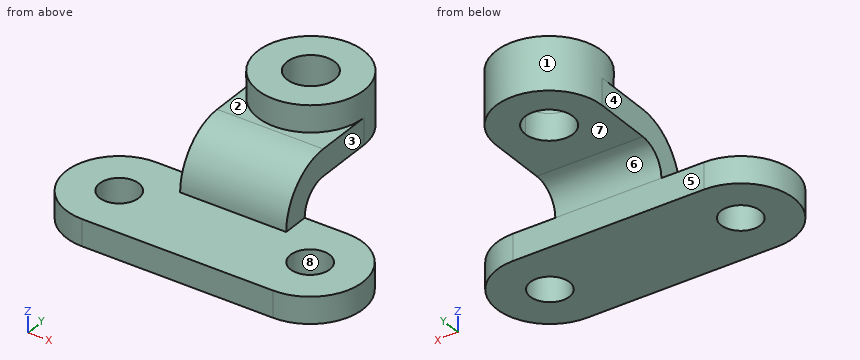
```python
from build123d import *
from build123d.topology import SkipClean

# Parameters (mm, degrees)
SKETCH1_R           = 18.5
BOSS_EXTRUDE1_DEPTH = 25
BOSS_EXTRUDE2_START = 100
SKETCH1_3_R         = 50
SKETCH1_3_R_2       = 22.5
BOSS_EXTRUDE2_DEPTH = 50
BOSS_EXTRUDE3_DEPTH = 50
CUT_EXTRUDE1_DEPTH  = 241.052077683


with BuildPart() as part:
    # Sketch1 → Boss-Extrude1 (new body)
    with BuildSketch(Plane.XY):
        with BuildLine():
            Line((-90, -50), (90, -50))
            ThreePointArc((90, -50), (140, 0), (90, 50))
            Line((90, 50), (-90, 50))
            ThreePointArc((-90, 50), (-140, 0), (-90, -50))
        make_face()
        with Locations((-90, 0)):
            Circle(SKETCH1_R, mode=Mode.SUBTRACT)
        with Locations((90, 0)):
            Circle(SKETCH1_R, mode=Mode.SUBTRACT)
    extrude(amount=BOSS_EXTRUDE1_DEPTH)



with BuildPart() as body_2:
    # Sketch1<3> → Boss-Extrude2 (new body)
    with BuildSketch(Plane.XY.offset(BOSS_EXTRUDE2_START)):
        with Locations((0, 130)):
            Circle(SKETCH1_3_R)
        with Locations((0, 130)):
            Circle(SKETCH1_3_R_2, mode=Mode.SUBTRACT)
    extrude(amount=-BOSS_EXTRUDE2_DEPTH)


with BuildPart() as part_1:
    add(part.part)

    add(body_2.part)  # Boss-Extrude3 merges body 2
    # Sketch2 → Boss-Extrude3 (add, symmetric)
    with BuildSketch(Plane(origin=(0, 0, 0), x_dir=(0, 0, -1), z_dir=(1, 0, 0))):
        with BuildLine():
            Line((-50, 130), (-50, 75))
            ThreePointArc((-50, 75), (-42.67766953, 57.32233047), (-25, 50))
            Line((-25, 50), (-12.5, 50))
            Line((-12.5, 50), (-12.5, 25))
            Line((-12.5, 25), (-25, 25))
            ThreePointArc((-25, 25), (-60.355339059, 39.644660941), (-75, 75))
            Line((-75, 75), (-75, 130))
            Line((-75, 130), (-50, 130))
        make_face()
    extrude(amount=BOSS_EXTRUDE3_DEPTH, both=True)

    # Sketch3 → Cut-Extrude1 (cut, through all)
    with SkipClean():  # the faces are left unmerged after this step: merging them gives an invalid solid
        with BuildSketch(Plane.XY.offset(75)):
            with BuildLine():
                Line((22.5, 130), (-22.5, 130))
                ThreePointArc((-22.5, 130), (0, 107.5), (22.5, 130))
            make_face()
        extrude(amount=-CUT_EXTRUDE1_DEPTH, mode=Mode.SUBTRACT)
    add(part_1.part.scale(1), mode=Mode.REPLACE)  # the faces are merged on a copy


solid = part_1.part
```
Input: part model. Units: mm. Frame: model coordinates. Face numbers are marked on the shaded views. A direction names the side the tool comes from. Coordinates: 2 decimals unless noted, no trailing zeros. Write each loop counter-clockwise with the first axis right and the second up, starting at its lowest first coordinate (ties: lowest second). Pieces come first, ordered by that corner, then holes. Notation, with made-up numbers: M -30,17.5 L 12,17.5 A34 ccw 12,48.5 Z; hole C 43.25,54.25 d5. An arc over 180 degrees is marked long. Use one line per item in the form item = value.
Q1. Section A-A (y = 0). Return loops of the section in (x, z).
Answer below:
outline = M -140,0 L -108.5,0 L -108.5,25 L -140,25 Z; M -71.5,0 L 71.5,0 L 71.5,25 L -71.5,25 Z; M 108.5,0 L 140,0 L 140,25 L 108.5,25 Z
Q2. Draft query along Y for the marked faces 6, 7 and 8. Return one class per face: released by +Y, released by -Y, zero draft, split by the parting line, or undercut.
Answer below:
face_6 = released by +Y
face_7 = zero draft
face_8 = undercut
Q3. First-contact query: pin 1 (7.5 mm diameter, centred on x = 41.5, z = 11.5, fed in from +Y); pin 2 (15 mm diameter, centred on y = 63, z = 40.5, fed in from -X); pin 3 (4 mm diameter, centred on x = 31, y = 137, fed in from -Z); pin 4 (15 mm diameter, centred on y = 99.5, z = 39.5, fed in from +X). Flat tips, straight axial feed; report the tip coordinate or a pass-through.
Answer below:
pin_1 = 50
pin_2 = -50
pin_3 = 50
pin_4 = through
Q4. Set-up query: the marked faces 1, 2, 3, 4 and 5. Return all of +Z, -Z, +X, -X, +Y, -Y with unobstructed straight access to the full face (end or side cutting, diameter ignored); none if empty.
Answer below:
face_1 = +Z
face_2 = +Z, -Y
face_3 = +Z, +X, +Y, -Y
face_4 = +Z, -X, +Y, -Y
face_5 = -Z, +X, -X, +Y
Q5. Material intervals for probe 1 along Y at (x, z) = (-90, 19.5); probe 2 along X at (y, z) = (130, 88); probe 3 along Z at (x, y) = (55.5, -18), sorted ascending. Write a range as from..to.
Answer below:
probe_1 = -50..-18.5, 18.5..50
probe_2 = -50..-22.5, 22.5..50
probe_3 = 0..25
Q6. Section C-C (z = 18). Return loops of the section in (x, y).
Answer below:
outline = M -90,-50 L 90,-50 A50 ccw 90,50 L -90,50 A50 ccw Z; hole C -90,0 d37; hole C 90,0 d37
Q7. Section D-D (z = 63.5). Return loops of the section in (x, y).
Answer below:
outline = M -50,43.1 L 50,43.1 L 50,130 A50 ccw -50,130 Z; hole C 0,130 d45
Q8. Section B-B (x = 0). Return loops of the section in (y, z), plus the area to 3 significant figures.
Answer below:
outline = M -50,0 L 50,0 L 50,25 A25 cw 75,50 L 107.5,50 L 107.5,100 L 80,100 L 80,75 L 75,75 A50 ccw 25,25 L -50,25 Z; M 152.5,50 L 180,50 L 180,100 L 152.5,100 Z
area = 6,850 mm²
